Could you check a few things on this model? Use its own coordinates, in mm. A direction names the side the tool comes from. Give positions to 0.01 mm unless a question says otherwise; leave off trailing zeros. Order: outer loops, then holes, each group sorted by start corner. A loop starts at its lowest first (then second) coordinate and runs counter-clockwise, first axis right, second up. Notation, with made-up numbers: (78.25, 75.5) - (133.25, 75.5) arc R21 ccw to (133.25, 81.5) - close; hole circle Ø8 at (14.25, -20). An arc over 180 degrees is marked (long way). Put each result on its own line as item: value.
from build123d import *

# Parameters (mm, degrees)
ESQUISSE1_W             = 70
ESQUISSE1_H             = 9
ESQUISSE1_R             = 1.8
BOSS_EXTRU_1_DEPTH      = 8
ESQUISSE2_R             = 2
ENL_V_MAT_EXTRU_1_DEPTH = 10
ESQUISSE3_R             = 2
BOSS_EXTRU_2_DEPTH      = 9
ESQUISSE4_W             = 5
ESQUISSE4_H             = 48.9
ENL_V_MAT_EXTRU_2_DEPTH = 10
ESQUISSE5_W             = 10
ESQUISSE5_H             = 9
ESQUISSE5_R             = 1.8
BOSS_EXTRU_3_DEPTH      = 7


with BuildPart() as part:
    # Esquisse1 → Boss.-Extru.1 (new body)
    with BuildSketch(Plane.XY):
        with Locations((35, 4.5)):
            Rectangle(ESQUISSE1_W, ESQUISSE1_H)
        with Locations((10, 4.5)):
            Circle(ESQUISSE1_R, mode=Mode.SUBTRACT)
        with Locations((60, 4.5)):
            Circle(ESQUISSE1_R, mode=Mode.SUBTRACT)
    extrude(amount=BOSS_EXTRU_1_DEPTH)

    # Esquisse2 → Enlèv. mat.-Extru.1 (cut)
    with BuildSketch(Plane.XZ):
        with Locations((30, 3.85)):
            Circle(ESQUISSE2_R)
        with Locations((40, 3.85)):
            Circle(ESQUISSE2_R)
    extrude(amount=-ENL_V_MAT_EXTRU_1_DEPTH, mode=Mode.SUBTRACT)

    # Esquisse3 → Boss.-Extru.2 (add)
    with BuildSketch(Plane(origin=(0, 9, 0), x_dir=(1, 0, 0), z_dir=(0, 1, 0))):
        Polygon((50, 0), (55, 0), (55, 48.9), (20, 48.9), (20, 0), (25, 0), (25, 40.9), (50, 40.9), align=None)
        with Locations(Location((30, 44.75, 0), (0, 0, 180))):
            Circle(ESQUISSE3_R, mode=Mode.SUBTRACT)
        with Locations(Location((40, 44.75, 0), (0, 0, 180))):
            Circle(ESQUISSE3_R, mode=Mode.SUBTRACT)
    extrude(amount=-BOSS_EXTRU_2_DEPTH)

    # Esquisse4 → Enlèv. mat.-Extru.2 (cut)
    with BuildSketch(Plane(origin=(0, 9, 0), x_dir=(1, 0, 0), z_dir=(0, 1, 0))):
        with Locations((52.5, 24.45)):
            Rectangle(ESQUISSE4_W, ESQUISSE4_H)
    extrude(amount=-ENL_V_MAT_EXTRU_2_DEPTH, mode=Mode.SUBTRACT)

    # Esquisse5 → Boss.-Extru.3 (add)
    with BuildSketch(Plane(origin=(50, 0, 0), x_dir=(0, 0, -1), z_dir=(1, 0, 0))):
        with Locations((53.9, 4.5)):
            Rectangle(ESQUISSE5_W, ESQUISSE5_H)
        with Locations(Location((53.9, 4.5, 0), (0, 0, 90))):
            Circle(ESQUISSE5_R, mode=Mode.SUBTRACT)
    extrude(amount=-BOSS_EXTRU_3_DEPTH)


solid = part.part
1) Suppose I cut it at A-A, the plane x = 45. List the corners of the cut face in (y, z) for me.
Filled in:
outline: (0, -58.9) - (9, -58.9) - (9, -40.9) - (0, -40.9) - close; (0, 0) - (9, 0) - (9, 8) - (0, 8) - close; hole circle Ø3.6 at (4.5, -53.9)
2) We'd pull the mould along X, two halves only. Please class faces 1 (the flat face through (50, 5, -50)), 2 (the cylindrical face through (8.2, 4.58, 3.94)), 3 (the flat face through (43, 7, -54)): pulls with the +X half, pulls with the -X half, needs draft (parallel to the pull), parting line crosses it, or undercut.
Filled in:
face 1: pulls with the +X half
face 2: undercut
face 3: pulls with the -X half
3) Suppose I cut it at B-B, the plane y = 4.5. List the corners of the cut face in (x, z) for me, and give its area (3 significant figures).
Filled in:
outline: (0, 0) - (8.2, 0) - (8.2, 8) - (0, 8) - close; (11.8, 0) - (20, 0) - (20, -48.9) - (43, -48.9) - (43, -52.1) - (50, -52.1) - (50, -40.9) - (25, -40.9) - (25, 0) - (58.2, 0) - (58.2, 8) - (11.8, 8) - close; (43, -58.9) - (50, -58.9) - (50, -55.7) - (43, -55.7) - close; (61.8, 0) - (70, 0) - (70, 8) - (61.8, 8) - close; hole circle Ø4 at (30, -44.75); hole circle Ø4 at (30, 3.85); hole circle Ø4 at (40, -44.75); hole circle Ø4 at (40, 3.85)
area: 941 mm^2
4) I'm going to push flat-ended pins straight in: pin 1 (2.5 mm diameter, centred on x = 37, y = 2.5, fed in from -Z); pin 2 (1.5 mm diameter, centred on x = 61.5, y = 7, fed in from -Z); pin 3 (4 mm diameter, centred on y = 3, z = -48.5, fed in from -X); pin 4 (5 mm diameter, centred on x = 46, z = -0.5, fed in from -Y). Where does each tip first touch, or does it pass through?
Filled in:
pin 1: stops at z = -48.9
pin 2: stops at z = 0
pin 3: stops at x = 20
pin 4: stops at y = 0
5) Which directions (+Z, -Z, +X, -X, +Y, -Y) give clear straight access to the entire face, cutting with the end or side of a thin tool? Please do faces 4 (the flat face through (25, 5, -20)), 5 (the flat face through (10, 7, 0)), 6 (the flat face through (47, 4, -58.9)).
Filled in:
face 4: +X, +Y, -Y
face 5: -Z, -X, +Y, -Y
face 6: -Z, +X, -X, +Y, -Y
6) If I drill on line 1 (Z direction, x = 30, y = 2.5); line 2 (Z direction, x = 46.25, y = 4.5); line 3 (Z direction, x = 48, y = 3), over which ranges is the centre line in solid material (lowest first)? Write a range as [from, to].
Filled in:
line 1: z = [-48.9, -46.75], [-42.75, -40.9], [0, 1.85], [5.85, 8]
line 2: z = [-58.9, -55.7], [-52.1, -40.9], [0, 8]
line 3: z = [-58.9, -54.89], [-52.91, -40.9], [0, 8]
7) Suppose I cut it at D-D, the plane x = 26.5. List the corners of the cut face in (y, z) for me.
Filled in:
outline: (0, -48.9) - (9, -48.9) - (9, -40.9) - (0, -40.9) - close; (0, 0) - (9, 0) - (9, 8) - (0, 8) - close
8) Suppose I cut it at C-C, the plane z = 3.85. List the corners of the cut face in (x, y) for me, and give its area (3 significant figures).
Filled in:
outline: (0, 0) - (28, 0) - (28, 9) - (0, 9) - close; (32, 0) - (38, 0) - (38, 9) - (32, 9) - close; (42, 0) - (70, 0) - (70, 9) - (42, 9) - close; hole circle Ø3.6 at (10, 4.5); hole circle Ø3.6 at (60, 4.5)
area: 538 mm^2
